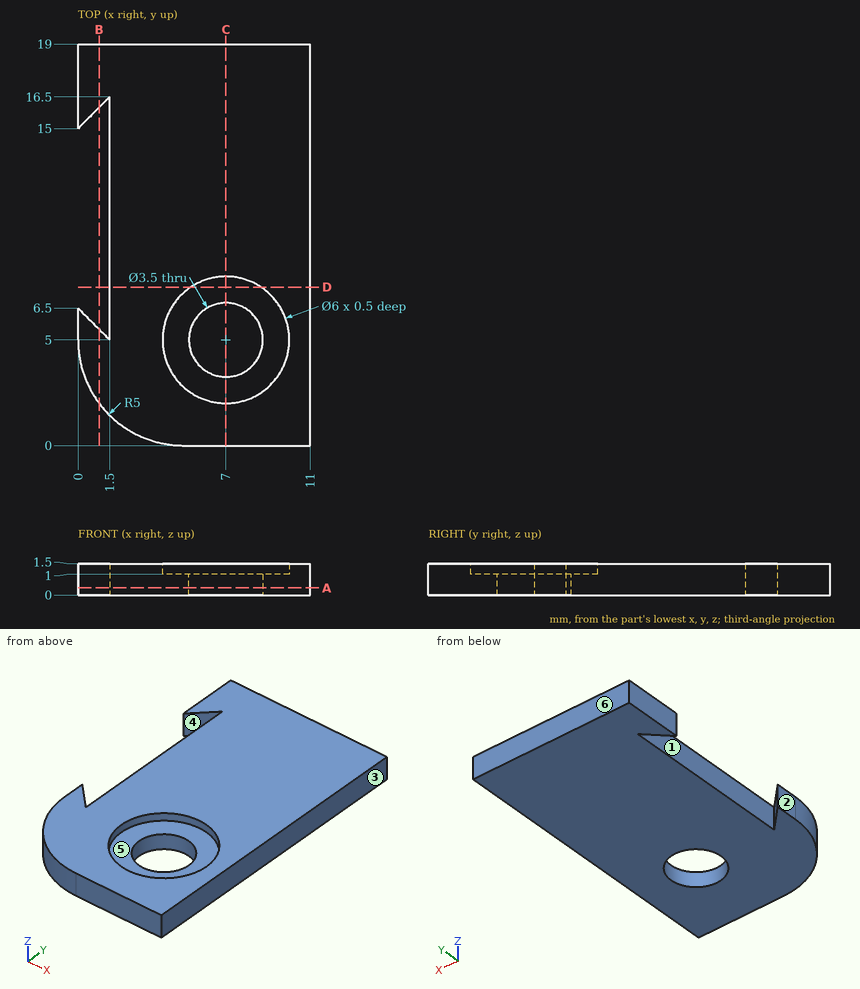
Input: dimensioned drawing with shaded views. Units: mm. Origin: part minimum x, y, z. A direction names the side the tool comes from. Give positions to 0.01 mm unless a question says otherwise; leave off trailing zeros. Write each loop counter-clockwise with the first axis right and the second up, starting at its lowest first coordinate (ties: lowest second). Pieces come first, ordered by that corner, then holes.
1. Pull-direction query (X, two-part tool) for the marked faces 1, 2 and 3; classes: +X half, -X half, draft (parallel to the pull), parting line (faces both ways), or undercut.
2. Access query for the marked faces 4, 5 and 6. Directions: +Z, -Z, +X, -X, +Y, -Y. A direction counts if a zero-diameter tool reaches every point of the face in a straight line with its end or side. Return the directions, or none.
3. Material intervals for line 1 along Y through (x, z) = (7, 0.75); line 2 along Y through (x, z) = (7, 1.3); line 3 along X through (y, z) = (5.75, 0.3), sorted ascending.
4. Section query B-B (x = 1). Return the cut outline in (y, z), then the cut area to 3 significant figures.
5. Section query D-D (y = 7.5). Return the cut outline in (x, z), then the cut area to 3 significant figures.
6. Section query A-A (z = 0.35). Return the cut outline in (x, y).
7. Section query C-C (x = 7). Return the cut outline in (y, z), then the cut area to 3 significant figures.
Output values:
1. face 1: undercut
1. face 2: -X half
1. face 3: +X half
2. face 4: +Z, -Z
2. face 5: +Z
2. face 6: +Z, -Z, +X, -X, +Y
3. line 1: y = 0 to 3.25, 6.75 to 19
3. line 2: y = 0 to 2, 8 to 19
3. line 3: x = 0 to 0.75, 1.5 to 5.42, 8.58 to 11
4. outline: (2, 0) - (5.5, 0) - (5.5, 1.5) - (2, 1.5) - close; (16, 0) - (19, 0) - (19, 1.5) - (16, 1.5) - close
4. area: 9.75 mm2
5. outline: (1.5, 0) - (11, 0) - (11, 1.5) - (8.66, 1.5) - (8.66, 1) - (5.34, 1) - (5.34, 1.5) - (1.5, 1.5) - close
5. area: 12.6 mm2
6. outline: (0, 5) arc R5 ccw to (5, 0) - (11, 0) - (11, 19) - (0, 19) - (0, 15) - (1.5, 16.5) - (1.5, 5) - (0, 6.5) - close; hole circle Ø3.5 at (7, 5)
7. outline: (0, 0) - (3.25, 0) - (3.25, 1) - (2, 1) - (2, 1.5) - (0, 1.5) - close; (6.75, 0) - (19, 0) - (19, 1.5) - (8, 1.5) - (8, 1) - (6.75, 1) - close
7. area: 22.0 mm2
